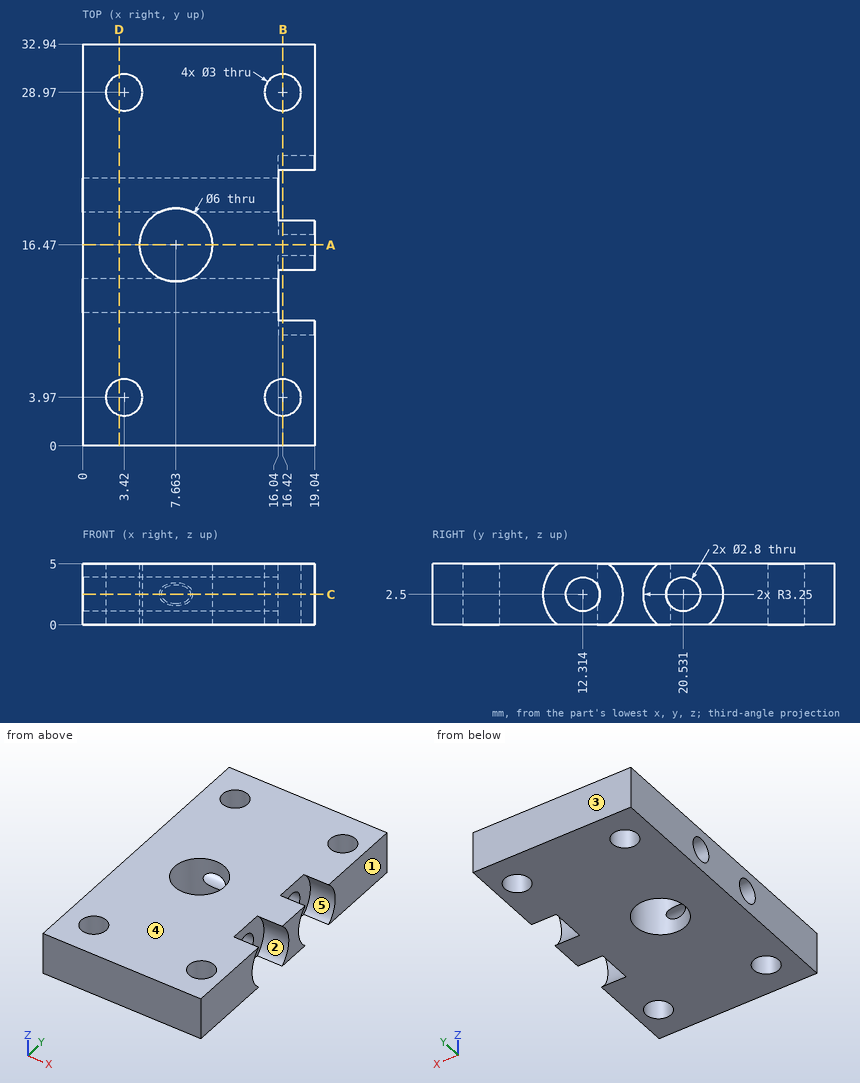
Job drawing, mm, ordinate dimensions from the low corner. One solid piece. A direction names the side the tool comes from. Coordinates: 2 decimals unless noted, no trailing zeros. Order: outer loops, then holes, each group sorted by start corner. A loop starts at its lowest first (then second) coordinate and runs counter-clockwise, first axis right, second up. Notation, with made-up numbers: (-37, -32) - (-19, -32) arc R14 cw to (-19, -22) - close; hole circle Ø2 at (52.25, 89). An arc over 180 degrees is marked (long way). Write each question's results on one line, items separated by ' | '. Start each with the question number.
Item 1: Flat gauge pin, fed straight in: pin 1 (1.5 mm diameter, centred on y = 10.5, z = 1, fed in from +X). Where does the tip first touch, or does it go through?
Item 2: Wall check: probe 1 along Y at (x, z) = (11, 2.65) (1 decimal); probe 2 along Y at (x, z) = (16.5, 2.3) (1 decimal); probe 3 along Y at (x, z) = (16.5, 4.3) (1 decimal). Give the ranges that are in metal, low to high. Write a range as [from, to].
Item 3: Band-saw the part on B-B on x = 16.42. State how many separate pieces and enclosed holes the cut face has.
Item 4: Band-saw the part on D-D on x = 3. Write the cut outline in (y, z), and give its area (3 significant figures).
Item 5: Band-saw the part on A-A on y = 16.47. Write the cut outline in (x, z), and give its area (3 significant figures).
Item 6: Band-saw the part on C-C on z = 2.5. Write the cut outline in (x, y), and give its area (3 significant figures).
Item 7: Tool access for the marked faces 1 and 2: list every direction of +Z, -Z, +X, -X, +Y, -Y with a clear straight run to the whole face (end or side of a thin tool).
Item 8: Mould opens along Y. For the marked faces 3, 4 and 5 say: released by +Y, released by -Y, zero draft, split by the parting line, or undercut.
Numbers:
1) pin 1: x = 16.04
2) probe 1: [0, 10.9], [13.7, 19.1], [21.9, 32.9] | probe 2: [0, 2.5], [5.5, 9.1], [15.6, 17.3], [23.8, 27.5], [30.5, 32.9] | probe 3: [0, 2.5], [5.5, 9.6], [15, 17.8], [23.2, 27.5], [30.5, 32.9]
3) separate pieces: 5 | enclosed holes: 0
4) outline: (0, 0) - (2.53, 0) - (2.53, 5) - (0, 5) - close; (5.41, 0) - (27.53, 0) - (27.53, 5) - (5.41, 5) - close; (30.41, 0) - (32.94, 0) - (32.94, 5) - (30.41, 5) - close; hole circle Ø2.8 at (12.31, 2.5); hole circle Ø2.8 at (20.53, 2.5) | area: 124 mm^2
5) outline: (0, 0) - (4.66, 0) - (4.66, 5) - (0, 5) - close; (10.66, 0) - (19.04, 0) - (19.04, 5) - (10.66, 5) - close | area: 65.2 mm^2
6) outline: (0, 0) - (19.04, 0) - (19.04, 9.06) - (16.04, 9.06) - (16.04, 10.91) - (0, 10.91) - close; (0, 13.71) - (6.48, 13.71) arc R3 cw to (6.28, 19.13) - (0, 19.13) - close; (0, 21.93) - (16.04, 21.93) - (16.04, 23.78) - (19.04, 23.78) - (19.04, 32.94) - (0, 32.94) - close; (8.85, 13.71) - (16.04, 13.71) - (16.04, 15.56) - (19.04, 15.56) - (19.04, 17.28) - (16.04, 17.28) - (16.04, 19.13) - (9.05, 19.13) arc R3 cw to start; hole circle Ø3 at (3.42, 3.97); hole circle Ø3 at (3.42, 28.97); hole circle Ø3 at (16.42, 3.97); hole circle Ø3 at (16.42, 28.97) | area: 443 mm^2
7) face 1: +Z, -Z, +X, +Y, -Y | face 2: +X
8) face 3: released by +Y | face 4: zero draft | face 5: undercut
